Design review of the part shown in the three views and the two pictorial views. Dimensions are in mm from the part's minimum x, y and z. A direction names the side the tool comes from. Coordinates: 2 decimals unless noted, no trailing zeros. Loops run counter-clockwise (first coordinate to the right, second up) from the corner with the lowest first, then second, coordinate; pieces in that order, holes last. Notation, with made-up numbers: (-34, 15.25) -> (20, 15.25) arc R19 ccw to (20, 48.25) -> close; hole circle Ø1 at (37.25, 28.5). An arc over 180 degrees is marked (long way). One line per item, written item: value. Start each with the question number.
1. Machinability: for the marked faces 1, 2 and 3, which of the approach directions +Z, -Z, +X, -X, +Y, -Y give a long, thin tool a straight path to every point of the face, cutting with its end or side? Answer none if there is none.
2. Insertion check: pin 1 (5.5 mm diameter, centred on x = 45.5, z = 28.5, fed in from -Y); pin 2 (7.5 mm diameter, centred on x = 33, y = 15, fed in from +Z); pin 3 (5 mm diameter, centred on x = 20.5, z = 48, fed in from +Y); pin 4 (6 mm diameter, centred on y = 25, z = 5.75, fed in from -X). Each pin has a flat end and moves straight along its axis. Give the tip position at first contact, or say it passes through.
3. Add section C-C on x = 36.5. Write out the cut boundary in (y, z), plus the area to 4 significant figures.
4. Add section A-A on z = 48. Write out the cut boundary in (x, y).
5. Add section B-B on y = 25. Write out the cut boundary in (x, z).
6. For probe 1 along Z at (x, y) = (20, 2); probe 2 along Y at (x, z) = (45, 5); probe 3 along Y at (x, z) = (28, 36.5), list the stretches that pass through material, from the lowest coordinate up.
7. Add section D-D on z = 42. Write out the cut boundary in (x, y).
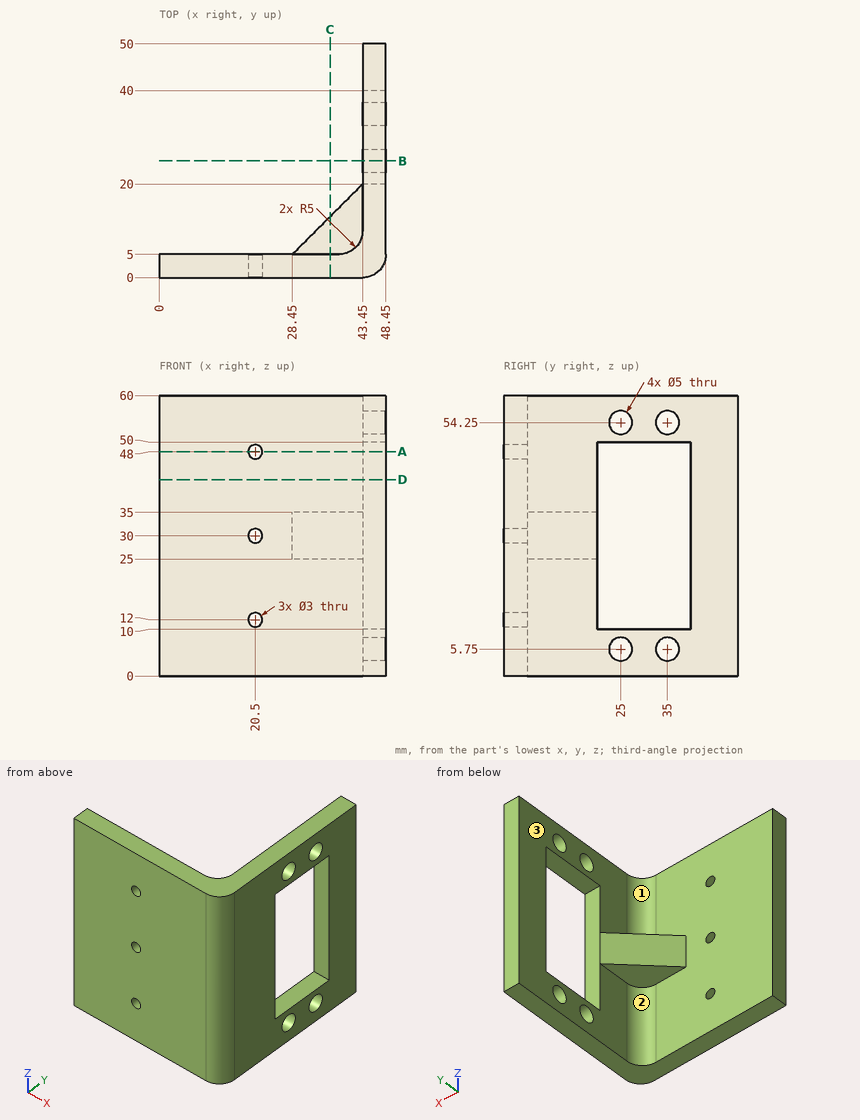
Worked answers:
1. face 1: +Z, -X, +Y
1. face 2: -Z, -X, +Y
1. face 3: -X, +Y
2. pin 1: stops at y = 0
2. pin 2: passes through
2. pin 3: stops at y = 5
2. pin 4: stops at x = 43.45
3. outline: (0, 0) -> (5, 0) -> (5, 25) -> (13.05, 25) -> (13.05, 35) -> (5, 35) -> (5, 60) -> (0, 60) -> close
3. area: 380.5 mm²
4. outline: (0, 0) -> (19, 0) -> (19, 5) -> (0, 5) -> close; (22, 0) -> (43.45, 0) arc R5 ccw to (48.45, 5) -> (48.45, 20) -> (43.45, 20) -> (43.45, 10) arc R5 cw to (38.45, 5) -> (22, 5) -> close; (43.45, 40) -> (48.45, 40) -> (48.45, 50) -> (43.45, 50) -> close
5. outline: (43.45, 0) -> (48.45, 0) -> (48.45, 3.25) -> (43.45, 3.25) -> close; (43.45, 8.25) -> (48.45, 8.25) -> (48.45, 10) -> (43.45, 10) -> close; (43.45, 50) -> (48.45, 50) -> (48.45, 51.75) -> (43.45, 51.75) -> close; (43.45, 56.75) -> (48.45, 56.75) -> (48.45, 60) -> (43.45, 60) -> close
6. probe 1: z = 0 to 10.59, 13.41 to 28.59, 31.41 to 46.59, 49.41 to 60
6. probe 2: y = 0.25 to 22.62, 27.38 to 32.62, 37.38 to 50
6. probe 3: y = 0 to 5
7. outline: (0, 0) -> (43.45, 0) arc R5 ccw to (48.45, 5) -> (48.45, 20) -> (43.45, 20) -> (43.45, 10) arc R5 cw to (38.45, 5) -> (0, 5) -> close; (43.45, 40) -> (48.45, 40) -> (48.45, 50) -> (43.45, 50) -> close
